from build123d import *

# Parameters (mm, degrees)
SKETCH_1_R          = 7
SKETCH_1_R_2        = 5.5
EXTRUDE_1_DEPTH     = 45
SKETCH_2_R          = 11.5
SKETCH_2_R_2        = 6.5
EXTRUDE_2_DEPTH     = 2
SKETCH_3_R          = 9
SKETCH_3_R_2        = 7.5
EXTRUDE_3_DEPTH     = 4.5
CHAMFER_1_SIZE      = 1.5
CUT_EXTRUDE_1_REACH = 62.237
SKETCH_5_W          = 1
SKETCH_5_H          = 5.956385966


with BuildPart() as part:
    # 草图1 → 凸台-拉伸1 (new body)
    with BuildSketch(Plane.XY):
        with Locations(Location((0, 0, 0), (0, 0, 180))):
            Circle(SKETCH_1_R)
        with Locations(Location((0, 0, 0), (0, 0, 180))):
            Circle(SKETCH_1_R_2, mode=Mode.SUBTRACT)
    extrude(amount=EXTRUDE_1_DEPTH)

    # 草图2 → 凸台-拉伸2 (add)
    with BuildSketch(Plane.XY.offset(45)):
        Circle(SKETCH_2_R)
        Circle(SKETCH_2_R_2, mode=Mode.SUBTRACT)
    extrude_2 = extrude(amount=EXTRUDE_2_DEPTH)

    # 草图3 → 凸台-拉伸3 (add)
    with BuildSketch(Plane.XY.offset(47)):
        Circle(SKETCH_3_R)
        Circle(SKETCH_3_R_2, mode=Mode.SUBTRACT)
    extrude_3 = extrude(amount=EXTRUDE_3_DEPTH)

    # 镜向16: 凸台-拉伸2, 凸台-拉伸3 across plane
    add(extrude_2.mirror(Plane(origin=(0, 0, 22.5), x_dir=(1, 0, 0), z_dir=(0, 0, -1))))
    add(extrude_3.mirror(Plane(origin=(0, 0, 22.5), x_dir=(1, 0, 0), z_dir=(0, 0, -1))))

    # 倒角1
    # the kernel refuses this chamfer: 1.5 mm, written as the material it adds along each edge
    with BuildSketch(Plane(origin=(0, 0, 45), x_dir=(1, 0, 0), z_dir=(0, -1, 0))) as chamfer_1_piece_1_section:
        Polygon((6.5, CHAMFER_1_SIZE), (6.5 - CHAMFER_1_SIZE, 0), (6.5, 0), align=None)
    chamfer_1_piece_1 = revolve(axis=Axis((0, 0, 45), (0, 0, 1)), mode=Mode.PRIVATE)
    chamfer_1_piece_1 = chamfer_1_piece_1 - Plane(origin=(0, 0, 45.996711571), x_dir=(-1, 0, 0), z_dir=(0, 0, -1)) * Cylinder(5.5, 26, mode=Mode.PRIVATE)
    add(chamfer_1_piece_1)
    with BuildSketch(Plane(origin=(0, 0, 0), x_dir=(1, 0, 0), z_dir=(0, -1, 0))) as chamfer_1_piece_2_section:
        Polygon((6.5, -CHAMFER_1_SIZE), (6.5 - CHAMFER_1_SIZE, 0), (6.5, 0), align=None)
    chamfer_1_piece_2 = revolve(axis=Axis((0, 0, 0), (0, 0, 1)), mode=Mode.PRIVATE)
    chamfer_1_piece_2 = chamfer_1_piece_2 - Plane(origin=(0, 0, -0.996711571), x_dir=(-1, 0, 0), z_dir=(0, 0, -1)) * Cylinder(5.5, 26, mode=Mode.PRIVATE)
    add(chamfer_1_piece_2)

    # 切除-拉伸1: up to this face of the body (flat: up to its plane)
    cut_extrude_1_end = Plane(part.part.faces().sort_by_distance((-11.174730881, 0, 0))[0])
    # 草图5 → 切除-拉伸1 (cut, up to the picked face)
    with BuildSketch(Plane(origin=(0, 0, -6.5), x_dir=(-1, 0, 0), z_dir=(0, 0, -1)), mode=Mode.PRIVATE) as cut_extrude_1_sk1:
        with Locations((0, 9.978192983)):
            Rectangle(SKETCH_5_W, SKETCH_5_H)
    cut_extrude_1_tool1 = split(extrude(cut_extrude_1_sk1.sketch, amount=-CUT_EXTRUDE_1_REACH, mode=Mode.PRIVATE), bisect_by=cut_extrude_1_end, keep=Keep.BOTH, mode=Mode.PRIVATE)
    add(cut_extrude_1_tool1.solids().sort_by(Axis((0, 9.978193, -6.5), (0, 0, 1)))[0], mode=Mode.SUBTRACT)


solid = part.part
CAD build for the part. Positions are in the model's coordinates, mm. A direction names the side the tool comes from. Give positions to 0.01 mm unless a question says otherwise; leave off trailing zeros. Write each loop counter-clockwise with the first axis right and the second up, starting at its lowest first coordinate (ties: lowest second). Pieces come first, ordered by that corner, then holes. Notation, with made-up numbers: (-5, -30.75) - (23, -30.75) arc R22 cw to (23, 7.25) - close; hole circle Ø9 at (61, 48). An arc over 180 degrees is marked (long way). Answer as CSV lines item,"result".
Q1. Pull direction Z, two halves, no side cores. Call faces 5 (the face through (0, -8, 0)), 6 (the face through (-7.493, 0.33, 49.218)), 7 (the face through (-6, -5, -6.5)), 8 (the face through (-6.466, 2.681, 22.185)): released by +Z, released by -Z, zero draft, split by the parting line, or undercut.
Result set:
face 5,"undercut"
face 6,"zero draft"
face 7,"released by -Z"
face 8,"undercut"
Q2. Band-saw the part on A-A (z = 16.5). Give the cut face in (x, y).
Result set:
outline,"circle Ø14 at (0, 0); hole circle Ø11 at (0, 0)"
Q3. 3-axis set-ups, long thin cutter, end or side, ignore diameter. For faces 1 (the face through (-6, 3, 47)), 2 (the face through (-0.5, 8.7, -2.6)), 3 (the face through (-5.158, -3.955, -1.746)), 4 (the face through (0, -8, 45)): which of +Z, -Z, +X, -X, +Y, -Y reach the whole face in a straight line?
Result set:
face 1,"+Z"
face 2,"-Z, +Y"
face 3,"-Z"
face 4,"none"
Q4. Flat gauge pins, fed straight in: pin 1 Ø3 at (y, z) = (0, 25.5) entering from -X; pin 2 Ø8 at (y, z) = (7.5, 18) entering from -X; pin 3 Ø12 at (x, y) = (0, -1) entering from +Z. Where does each tip first touch, or does it go through?
Result set:
pin 1,"x = -7"
pin 2,"x = -6.06"
pin 3,"z = 47"
Q5. Drill centre lines: line 1 (Y direction, x = 0, z = -1.75); line 2 (Z direction, x = 10, y = -0.5); line 3 (Y direction, x = 0, z = 48.4). Where is each one in solid material? Low to high. Write a range as from..to.
Result set:
line 1,"-11.5..-6.5, 6.5..7"
line 2,"-2..0, 45..47"
line 3,"-9..-7.5, 7.5..9"
